Can you work these out from the model? Positions are in its coordinate system, mm. Face numbers are marked on the shaded views. Round coordinates to 2 decimals unless told otherwise and drop trailing zeros. Loops run counter-clockwise (first coordinate to the right, second up) from the corner with the lowest first, then second, coordinate; pieces in that order, holes last.
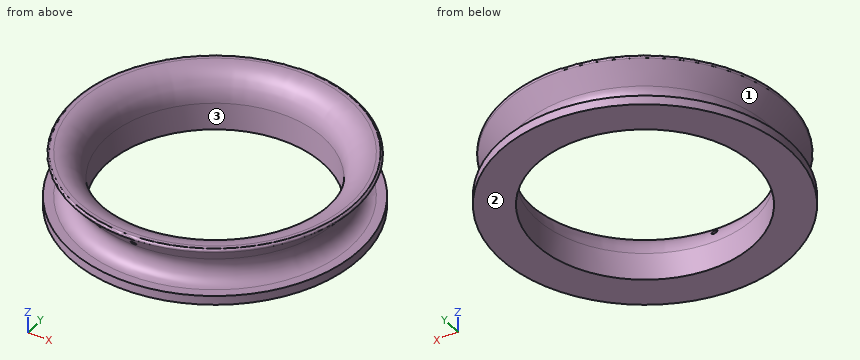
```python
from build123d import *

# Parameters (mm, degrees)
F3_R     = 1.5
F4_DEPTH = 80.001


with BuildPart() as f2:
    # F0 (on Front) → F2 (revolve)
    with BuildSketch(Plane.XZ):
        with BuildLine():
            Line((-80, 5), (-80, 0))
            Line((-80, 0), (-60, 0))
            Line((-60, 0), (-60, 15))
            ThreePointArc((-60, 15), (-64.393398, 25.606602), (-75, 30))
            Line((-75, 30), (-77, 30))
            ThreePointArc((-77, 30), (-77.947917, 29.318518), (-77.603858, 28.202908))
            Line((-77.603858, 28.202908), (-69, 18.291503))
            ThreePointArc((-69, 18.291503), (-67.708497, 9.708497), (-75, 5))
            Line((-75, 5), (-80, 5))
        make_face()
    revolve(axis=Axis((0, 0, 28.539639), (0, 0, 1)))

    # F3 (on Front) → F4 (cut, through all)
    with BuildSketch(Plane.XZ):
        with Locations((0, 22)):
            Circle(F3_R)
    extrude(amount=F4_DEPTH, mode=Mode.SUBTRACT)


solid = f2.part
```
(1) If I drill on line 1 (X direction, y = 0, z = 4.25); line 2 (X direction, y = -18, z = 2); line 3 (Z direction, x = 22, y = 71), over which ranges is the centre line in solid material (lowest first)?
(2) Suppose I cut it at B-B (z = 2). Write out the boundary of the cut face in (x, y), then the cut area to 3 significant figures.
(3) For pin 1 (2 mm diameter, centred on x = -16.5, z = 3.5, fed in from -Y); pin 2 (3 mm diameter, centred on y = 54, z = 11, fed in from +X); pin 3 (3 mm diameter, centred on x = -47, z = 13, fed in from -Y); pin 4 (6 mm diameter, centred on x = 18, y = -53.5, fed in from +Z), each with a flat end and sliding along its axis, tell me the tip position at first contact or that it passes through.
(4) Suppose I cut it at A-A (y = 0). Write out the boundary of the cut face in (x, z).
(5) Suppose I cut it at C-C (z = 12). Write out the boundary of the cut face in (x, y).
(6) We'd pull the mould along Y, two halves only. Please class the marked faces 1, 2 and 3: released by +Y, released by -Y, zero draft, split by the parting line, or undercut.
Check result:
1. line 1: x = -80 to -60, 60 to 80
1. line 2: x = -77.95 to -57.24, 57.24 to 77.95
1. line 3: z = 0 to 5.03, 24.43 to 29.99
2. outline: circle Ø160 at (0, 0); hole circle Ø120 at (0, 0)
2. area: 8,800 mm2
3. pin 1: stops at y = -78.48
3. pin 2: stops at x = 42.17
3. pin 3: stops at y = -49.18
3. pin 4: passes through
4. outline: (-80, 0) - (-60, 0) - (-60, 15) arc R15 ccw to (-75, 30) - (-77, 30) arc R1 ccw to (-77.6, 28.2) - (-69, 18.29) arc R8 cw to (-75, 5) - (-80, 5) - close; (60, 0) - (80, 0) - (80, 5) - (75, 5) arc R8 cw to (69, 18.29) - (77.6, 28.2) arc R1 ccw to (77, 30) - (75, 30) arc R15 ccw to (60, 15) - close
5. outline: circle Ø134.13 at (0, 0); hole circle Ø120 at (0, 0)
6. face 1: split by the parting line
6. face 2: zero draft
6. face 3: undercut
